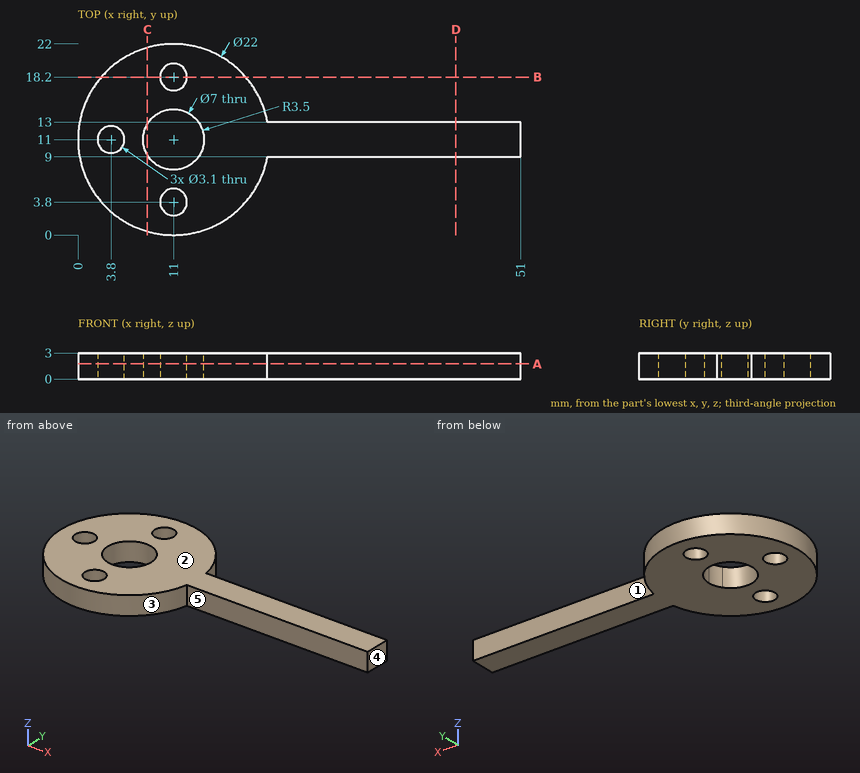
Can you work these out from the drawing? Everything is in mm from the part's minimum corner. A direction names the side the tool comes from. Give positions to 0.01 mm unless a question says otherwise; leave off trailing zeros. Loops run counter-clockwise (first coordinate to the right, second up) from the corner with the lowest first, then second, coordinate; pieces in that order, holes last. Notation, with made-up numbers: (56.5, 14.5) - (62.5, 14.5) arc R21 ccw to (62.5, 38.5) - close; hole circle Ø2 at (-37.75, 83.5). An arc over 180 degrees is marked (long way). Answer as a JSON object with one key per item and string values.
Q1. Imagine slicing it at A-A on z = 1.75. Write out the boundary of the cut face in (x, y), plus the area to 3 significant figures.
Geometry says:
{"outline": "(21.82, 9) - (51, 9) - (51, 13) - (21.82, 13) arc R11 ccw (long way) to start; hole circle Ø3.1 at (3.8, 11); hole circle Ø7 at (11, 11); hole circle Ø3.1 at (11, 3.8); hole circle Ø3.1 at (11, 18.2)", "area": "435 mm²"}
Q2. Imagine slicing it at C-C on x = 8. Write out the boundary of the cut face in (y, z), plus the area to 3 significant figures.
Geometry says:
{"outline": "(0.42, 0) - (9.2, 0) - (9.2, 3) - (0.42, 3) - close; (12.8, 0) - (21.58, 0) - (21.58, 3) - (12.8, 3) - close", "area": "52.7 mm²"}
Q3. Which directions (+Z, -Z, +X, -X, +Y, -Y) give clear straight access to the entire face, cutting with the end or side of a thin tool? Please do the marked faces 1 and 2.
Geometry says:
{"face 1": "+Z, -Z, +X, +Y", "face 2": "+Z, +X, -X, +Y, -Y"}
Q4. If we mould it in two halves opening along X, with no side actions, what happens to the marked faces 3, 4 and 5? For each: pulls with the +X half, pulls with the -X half, needs draft (parallel to the pull), parting line crosses it, or undercut.
Geometry says:
{"face 3": "parting line crosses it", "face 4": "pulls with the +X half", "face 5": "needs draft"}
Q5. Imagine slicing it at B-B on y = 18.2. Write out the boundary of the cut face in (x, z), plus the area to 3 significant figures.
Geometry says:
{"outline": "(2.68, 0) - (9.45, 0) - (9.45, 3) - (2.68, 3) - close; (12.55, 0) - (19.32, 0) - (19.32, 3) - (12.55, 3) - close", "area": "40.6 mm²"}
Q6. Will these pins go through, and if not, where does the flat tip stop? P1, Ø6.5, axis at x = 11, y = 11, coming from the -Z side; P2, Ø0.9, axis at x = 36.5, z = 2, coming from the +Y side; P3, Ø1.5, axis at x = 18, z = 2, coming from the +Y side.
Geometry says:
{"P1": "through", "P2": "y = 13", "P3": "y = 20.05"}
Q7. Imagine slicing it at D-D on x = 43.5. Write out the boundary of the cut face in (y, z).
Geometry says:
{"outline": "(9, 0) - (13, 0) - (13, 3) - (9, 3) - close"}
Q8. If I drill on L1, parallel to X at y = 11, z = 1.15; L2, parallel to Y at x = 36, z = 2.2; L3, parallel to X at y = 8, z = 0.2, over which ranges is the centre line in solid material (lowest first)?
Geometry says:
{"L1": "0 to 2.25, 5.35 to 7.5, 14.5 to 51", "L2": "9 to 13", "L3": "0.42 to 9.2, 12.8 to 21.58"}
